Build history of the part. All positions in model axes, mm. A direction names the side the tool comes from. Round coordinates to 2 decimals unless told otherwise and drop trailing zeros. Order: outer loops, then holes, each group sorted by start corner. A loop starts at its lowest first (then second) coordinate and runs counter-clockwise, first axis right, second up. Notation, with made-up numbers: M 64.5,-23.5 L 113.5,-23.5 A25 ccw 113.5,-2.5 Z; hole C 66,79 d5. An arc over 180 degrees is marked long. Use CSV: the item, a comma, the result in double quotes.
from build123d import *

# Parameters (mm, degrees)
SKIZZE1_W                       = 10
SKIZZE1_H                       = 10
SKIZZE1_R                       = 2.9
AUFSATZ_LINEAR_AUSTRAGEN3_DEPTH = 12
SKIZZE2_R                       = 3.95
SCHNITT_LINEAR_AUSTRAGEN1_DEPTH = 12
KREISMUSTER1_COUNT              = 12
VERRUNDUNG1_R                   = 5


with BuildPart() as part:
    # Skizze1 → Aufsatz-Linear austragen3 (new body)
    with BuildSketch(Plane.XY):
        with BuildLine():
            Line((-59.791303716, 5), (-59.791303716, -5))
            Line((-59.791303716, -5), (-45.727453461, -5))
            ThreePointArc((-45.727453461, -5), (-46, 0), (-45.727453461, 5))
            Line((-45.727453461, 5), (-59.791303716, 5))
        make_face()
        with BuildLine():
            ThreePointArc((-45.727453461, 5), (-46, 0), (-45.727453461, -5))
            Line((-45.727453461, -5), (-8.660254038, -5))
            ThreePointArc((-8.660254038, -5), (-10, 0), (-8.660254038, 5))
            Line((-8.660254038, 5), (-45.727453461, 5))
        make_face()
        with BuildLine():
            Line((8.660254038, -5), (45.727453461, -5))
            ThreePointArc((45.727453461, -5), (45.931812827, -2.503711326), (46, 0))
            ThreePointArc((46, 0), (45.931812827, 2.503711326), (45.727453461, 5))
            Line((45.727453461, 5), (8.660254038, 5))
            ThreePointArc((8.660254038, 5), (9.659258263, 2.588190451), (10, 0))
            ThreePointArc((10, 0), (9.659258263, -2.588190451), (8.660254038, -5))
        make_face()
        Rectangle(SKIZZE1_W, SKIZZE1_H)
        Circle(SKIZZE1_R, mode=Mode.SUBTRACT)
        with BuildLine():
            ThreePointArc((-8.660254038, 5), (-10, 0), (-8.660254038, -5))
            Line((-8.660254038, -5), (-5, -5))
            Line((-5, -5), (-5, 5))
            Line((-5, 5), (-8.660254038, 5))
        make_face()
        with BuildLine():
            ThreePointArc((-5, 8.660254038), (-7.071067812, 7.071067812), (-8.660254038, 5))
            Line((-8.660254038, 5), (-5, 5))
            Line((-5, 5), (-5, 8.660254038))
        make_face()
        with BuildLine():
            Line((-5, 8.660254038), (-5, 5))
            Line((-5, 5), (5, 5))
            Line((5, 5), (5, 8.660254038))
            ThreePointArc((5, 8.660254038), (0, 10), (-5, 8.660254038))
        make_face()
        with BuildLine():
            Line((5, 8.660254038), (5, 5))
            Line((5, 5), (8.660254038, 5))
            ThreePointArc((8.660254038, 5), (7.071067812, 7.071067812), (5, 8.660254038))
        make_face()
        with BuildLine():
            Line((5, 5), (5, -5))
            Line((5, -5), (8.660254038, -5))
            ThreePointArc((8.660254038, -5), (9.659258263, -2.588190451), (10, 0))
            ThreePointArc((10, 0), (9.659258263, 2.588190451), (8.660254038, 5))
            Line((8.660254038, 5), (5, 5))
        make_face()
        with BuildLine():
            Line((45.727453461, -5), (59.791303716, -5))
            Line((59.791303716, -5), (59.791303716, 5))
            Line((59.791303716, 5), (45.727453461, 5))
            ThreePointArc((45.727453461, 5), (45.931812827, 2.503711326), (46, 0))
            ThreePointArc((46, 0), (45.931812827, -2.503711326), (45.727453461, -5))
        make_face()
        with BuildLine():
            ThreePointArc((59.791303716, 5), (42.426406871, 42.426406871), (5, 59.791303716))
            Line((5, 59.791303716), (5, 45.727453461))
            ThreePointArc((5, 45.727453461), (32.526911935, 32.526911935), (45.727453461, 5))
            Line((45.727453461, 5), (59.791303716, 5))
        make_face()
        with BuildLine():
            Line((5, 59.791303716), (-5, 59.791303716))
            Line((-5, 59.791303716), (-5, 45.727453461))
            ThreePointArc((-5, 45.727453461), (0, 46), (5, 45.727453461))
            Line((5, 45.727453461), (5, 59.791303716))
        make_face()
        with BuildLine():
            ThreePointArc((-5, 59.791303716), (-42.426406871, 42.426406871), (-59.791303716, 5))
            Line((-59.791303716, 5), (-45.727453461, 5))
            ThreePointArc((-45.727453461, 5), (-32.526911935, 32.526911935), (-5, 45.727453461))
            Line((-5, 45.727453461), (-5, 59.791303716))
        make_face()
        with BuildLine():
            Line((-5, -8.660254038), (-5, -45.727453461))
            ThreePointArc((-5, -45.727453461), (0, -46), (5, -45.727453461))
            Line((5, -45.727453461), (5, -8.660254038))
            ThreePointArc((5, -8.660254038), (0, -10), (-5, -8.660254038))
        make_face()
        with BuildLine():
            ThreePointArc((5, 45.727453461), (0, 46), (-5, 45.727453461))
            Line((-5, 45.727453461), (-5, 8.660254038))
            ThreePointArc((-5, 8.660254038), (0, 10), (5, 8.660254038))
            Line((5, 8.660254038), (5, 45.727453461))
        make_face()
        with BuildLine():
            Line((-5, -5), (-8.660254038, -5))
            ThreePointArc((-8.660254038, -5), (-7.071067812, -7.071067812), (-5, -8.660254038))
            Line((-5, -8.660254038), (-5, -5))
        make_face()
        with BuildLine():
            Line((5, -5), (-5, -5))
            Line((-5, -5), (-5, -8.660254038))
            ThreePointArc((-5, -8.660254038), (0, -10), (5, -8.660254038))
            Line((5, -8.660254038), (5, -5))
        make_face()
        with BuildLine():
            Line((8.660254038, -5), (5, -5))
            Line((5, -5), (5, -8.660254038))
            ThreePointArc((5, -8.660254038), (7.071067812, -7.071067812), (8.660254038, -5))
        make_face()
        with BuildLine():
            Line((-45.727453461, -5), (-59.791303716, -5))
            ThreePointArc((-59.791303716, -5), (-42.426406871, -42.426406871), (-5, -59.791303716))
            Line((-5, -59.791303716), (-5, -45.727453461))
            ThreePointArc((-5, -45.727453461), (-32.526911935, -32.526911935), (-45.727453461, -5))
        make_face()
        with BuildLine():
            Line((-5, -45.727453461), (-5, -59.791303716))
            Line((-5, -59.791303716), (5, -59.791303716))
            Line((5, -59.791303716), (5, -45.727453461))
            ThreePointArc((5, -45.727453461), (0, -46), (-5, -45.727453461))
        make_face()
        with BuildLine():
            Line((5, -45.727453461), (5, -59.791303716))
            ThreePointArc((5, -59.791303716), (42.426406871, -42.426406871), (59.791303716, -5))
            Line((59.791303716, -5), (45.727453461, -5))
            ThreePointArc((45.727453461, -5), (32.526911935, -32.526911935), (5, -45.727453461))
        make_face()
    extrude(amount=AUFSATZ_LINEAR_AUSTRAGEN3_DEPTH)

    # Skizze2 → Schnitt-Linear austragen1 (cut)
    with BuildSketch(Plane.XY.offset(12)):
        with Locations((0, -53)):
            Circle(SKIZZE2_R)
    schnitt_linear_austragen1 = extrude(amount=-SCHNITT_LINEAR_AUSTRAGEN1_DEPTH, mode=Mode.SUBTRACT)

    # Kreismuster1: Schnitt-Linear austragen1 ×12 about axis
    kreismuster1_axis = Axis((0, 0, 0), (0, 0, 1))
    for i in range(1, KREISMUSTER1_COUNT):
        add(schnitt_linear_austragen1.rotate(kreismuster1_axis, i * 360 / KREISMUSTER1_COUNT), mode=Mode.SUBTRACT)

    # Verrundung1
    verrundung1_edges = [part.edges().sort_by_distance(p)[0] for p in [
        (-8.660254038, -5, 6),
        (-45.727453461, -5, 6),
        (-5, -45.727453461, 6),
        (-5, -8.660254038, 6),
        (-5, 45.727453461, 6),
        (-45.727453461, 5, 6),
        (-8.660254038, 5, 6),
        (-5, 8.660254038, 6),
        (45.727453461, 5, 6),
        (5, 45.727453461, 6),
        (5, 8.660254038, 6),
        (8.660254038, 5, 6),
        (5, -8.660254038, 6),
        (5, -45.727453461, 6),
        (45.727453461, -5, 6),
        (8.660254038, -5, 6),
    ]]
    fillet(verrundung1_edges, radius=VERRUNDUNG1_R)


solid = part.part
(1) Cut at A-A, the plane x = 0. Give the cut face in (y, z), and give its area (3 significant figures).
Answer block:
outline,"M -59.79,0 L -56.95,0 L -56.95,12 L -59.79,12 Z; M -49.05,0 L -2.9,0 L -2.9,12 L -49.05,12 Z; M 2.9,0 L 49.05,0 L 49.05,12 L 2.9,12 Z; M 56.95,0 L 59.79,0 L 59.79,12 L 56.95,12 Z"
area,"1,180 mm²"
(2) Wall check: line 1 (Y direction, x = 12.5, z = 8.5); line 2 (X direction, y = -45.5, z = 11.5); line 3 (X direction, y = -18, z = 8.75). Give the ranges that are in metal, low to high. Write a range as from..to.
Answer block:
line 1,"y = -58.68..-44.27, -5..5, 44.27..58.68"
line 2,"x = -39.11..-30.43, -22.57..22.57, 30.43..39.11"
line 3,"x = -57.24..-42.33, -5..5, 42.33..57.24"
(3) Cut at D-D, the plane x = 20. Give the cut face in (y, z), and give its area (3 significant figures).
Answer block:
outline,"M -56.57,0 L -41.42,0 L -41.42,12 L -56.57,12 Z; M -5,0 L 5,0 L 5,12 L -5,12 Z; M 41.42,0 L 56.57,0 L 56.57,12 L 41.42,12 Z"
area,"483 mm²"
(4) Two-plate mould, pull along X, no slides. Class faces 3 (the face through (-0.514, -49.084, 6.084)), 4 (the face through (-42.84, -42.01, 5.92)), 5 (the face through (42.01, -42.84, 5.92)), 6 (the face through (-1, -12, 0)): released by +X, released by -X, zero draft, split by the parting line, or undercut.
Answer block:
face 3,"undercut"
face 4,"released by -X"
face 5,"released by +X"
face 6,"zero draft"
(5) Drop flat-ended pins along their axis: pin 1 (7 mm diameter, centred on x = 45.9, y = -26.5, fed in from -Z); pin 2 (1 mm diameter, centred on x = -47.5, z = 4.5, fed in from -Y); pin 3 (6 mm diameter, centred on x = 30, z = 6, fed in from +Y); pin 4 (6 mm diameter, centred on y = 23, z = 6.5, fed in from +X). Give the stop position or say it passes through.
Answer block:
pin 1,"passes through"
pin 2,"stops at y = -37.3"
pin 3,"stops at y = 53.58"
pin 4,"stops at x = 56.57"
(6) Tool access for faces 1 (the face through (0, 59.791, 6)), 2 (the face through (32.77, -32.28, 5.92)): list every direction of +Z, -Z, +X, -X, +Y, -Y with a clear straight run to the whole face (end or side of a thin tool).
Answer block:
face 1,"+Z, -Z, +X, -X, +Y"
face 2,"+Z, -Z"
(7) Cut at C-C, the plane y = -26.5. Give the cut face in (x, z).
Answer block:
outline,"M -53.83,0 L -49.85,0 L -49.85,12 L -53.83,12 Z; M -41.95,0 L -37.6,0 L -37.6,12 L -41.95,12 Z; M -5,0 L 5,0 L 5,12 L -5,12 Z; M 37.6,0 L 41.95,0 L 41.95,12 L 37.6,12 Z; M 49.85,0 L 53.83,0 L 53.83,12 L 49.85,12 Z"
